from build123d import *

# Parameters (mm, degrees)
SKETCH4_W               = 63.691174053
SKETCH4_H               = 96.012068348
CUT_EXTRUDE3_DEPTH      = 86.451740766
CUT_EXTRUDE4_DEPTH      = 86.451740766
CUT_EXTRUDE4_DEPTH_BACK = 86.451740766
SKETCH6_R               = 1.65
CUT_EXTRUDE5_DEPTH      = 90.173515588
CUT_EXTRUDE5_DEPTH_BACK = 90.173515588
SKETCH7_R               = 1.65
SKETCH9_R               = 1.65
CUT_EXTRUDE7_DEPTH      = 5
BOSS_EXTRUDE4_START     = 27
SKETCH16_R              = 3.65
SKETCH16_R_2            = 1.65
BOSS_EXTRUDE4_DEPTH     = 3.9
BOSS_EXTRUDE6_START     = -16
SKETCH17_R              = 3.65
SKETCH17_R_2            = 1.65
BOSS_EXTRUDE6_DEPTH     = 3.9
BOSS_EXTRUDE7_START     = 4
SKETCH18_R              = 1.65
BOSS_EXTRUDE7_DEPTH     = 4
CUT_EXTRUDE8_DEPTH      = 0.2
SKETCH22_R              = 2.05
BOSS_EXTRUDE8_DEPTH     = 2
MIRROR2_COPY_1_SKETCH_R = 2.05
MIRROR2_COPY_1_DEPTH    = 2


with BuildPart() as part:
    # Sketch1 → Revolve1 (revolve)
    with BuildSketch(Plane(origin=(0, 0, 0), x_dir=(0, 0, -1), z_dir=(1, 0, 0)), mode=Mode.PRIVATE) as revolve1_sk:
        with BuildLine():
            Line((0, 12), (0, 11))
            Line((0, 11), (2, 11))
            Line((2, 11), (2, 10.5))
            ThreePointArc((2, 10.5), (3.464466094, 14.035533906), (7, 15.5))
            Line((7, 15.5), (12, 15.5))
            Line((12, 15.5), (75, 15.5))
            ThreePointArc((75, 15.5), (78.535533906, 14.035533906), (80, 10.5))
            Line((80, 10.5), (80, 0))
            Line((80, 0), (82, 0))
            Line((82, 0), (82, 12))
            ThreePointArc((82, 12), (80.535533906, 15.535533906), (77, 17))
            Line((77, 17), (5, 17))
            ThreePointArc((5, 17), (1.464466094, 15.535533906), (0, 12))
        make_face()
    revolve(revolve1_sk.sketch.rotate(Axis((0, 0, 0), (0, 0, -1)), 180), axis=Axis((0, 0, 0), (0, 0, -1)))

    # Sketch4 → Cut-Extrude3 (cut, through all)
    with BuildSketch(Plane(origin=(0, 0, 0), x_dir=(1, 0, 0), z_dir=(0, 1, 0))):
        with Locations((-0.095061454, 42.091351984)):
            Rectangle(SKETCH4_W, SKETCH4_H)
    extrude(amount=CUT_EXTRUDE3_DEPTH, mode=Mode.SUBTRACT)

    # Sketch6 → Cut-Extrude4 (cut, two sides: drawn at the far end of the back side and taken through both)
    with BuildSketch(Plane(origin=(0, 0, 0), x_dir=(0.7071067811865477, 0.7071067811865475, 0), z_dir=(-0.7071067811865475, 0.7071067811865477, 0)).offset(-CUT_EXTRUDE4_DEPTH_BACK)):
        with Locations(Location((0, 41, 0), (0, 0, 180))):
            Circle(SKETCH6_R)
    extrude(amount=CUT_EXTRUDE4_DEPTH + CUT_EXTRUDE4_DEPTH_BACK, mode=Mode.SUBTRACT)

    # Sketch7 → Cut-Extrude5 (cut, two sides: drawn at the far end of the back side and taken through both)
    with BuildSketch(Plane(origin=(7.778174593, 7.778174593, 0), x_dir=(0, 0, 1), z_dir=(-0.7071067811865438, -0.7071067811865512, 0)).offset(-CUT_EXTRUDE5_DEPTH_BACK)):
        with Locations(Location((-41, 0, 0), (0, 0, 270))):
            Circle(SKETCH7_R)
    extrude(amount=CUT_EXTRUDE5_DEPTH + CUT_EXTRUDE5_DEPTH_BACK, mode=Mode.SUBTRACT)

    # Sketch9 → Cut-Extrude7 (cut)
    with BuildSketch(Plane(origin=(0, 0, -82), x_dir=(-1, 0, 0), z_dir=(0, 0, -1))):
        with Locations(Location((0, -10, 0), (0, 0, 90))):
            Circle(SKETCH9_R)
    extrude(amount=-CUT_EXTRUDE7_DEPTH, mode=Mode.SUBTRACT)

    # Sketch16 → Boss-Extrude4 (add)
    with BuildSketch(Plane(origin=(7.778174593, 7.778174593, 0), x_dir=(0, 0, 1), z_dir=(-0.7071067811865438, -0.7071067811865512, 0)).offset(BOSS_EXTRUDE4_START)):
        with Locations(Location((-41, 0, 0), (0, 0, 90))):
            Circle(SKETCH16_R)
        with Locations(Location((-41, 0, 0), (0, 0, 270))):
            Circle(SKETCH16_R_2, mode=Mode.SUBTRACT)
    extrude(amount=BOSS_EXTRUDE4_DEPTH)

    # Sketch17 → Boss-Extrude6 (add)
    with BuildSketch(Plane(origin=(0, 0, 0), x_dir=(0.7071067811865477, 0.7071067811865475, 0), z_dir=(-0.7071067811865475, 0.7071067811865477, 0)).offset(BOSS_EXTRUDE6_START)):
        with Locations(Location((0, 41, 0), (0, 0, 180))):
            Circle(SKETCH17_R)
        with Locations(Location((0, 41, 0), (0, 0, 180))):
            Circle(SKETCH17_R_2, mode=Mode.SUBTRACT)
    extrude(amount=-BOSS_EXTRUDE6_DEPTH)

    # Sketch18 → Boss-Extrude7 (add)
    with BuildSketch(Plane(origin=(0, 0, -82), x_dir=(-1, 0, 0), z_dir=(0, 0, -1)).offset(BOSS_EXTRUDE7_START)):
        with BuildLine():
            Line((-4.806077942, -8.559024607), (-9, 0))
            Line((-9, 0), (-6.25, 0))
            ThreePointArc((-6.25, 0), (-5.298097039, -2.298097039), (-3, -3.25))
            Line((-3, -3.25), (3, -3.25))
            ThreePointArc((3, -3.25), (5.298097039, -2.298097039), (6.25, 0))
            Line((6.25, 0), (9, 0))
            Line((9, 0), (4.806077942, -8.559024607))
            ThreePointArc((4.806077942, -8.559024607), (4.337052511, -9.685379412), (4.008689498, -10.860469933))
            ThreePointArc((4.008689498, -10.860469933), (0, -14.1), (-4.008689498, -10.860469933))
            ThreePointArc((-4.008689498, -10.860469933), (-4.337052511, -9.685379412), (-4.806077942, -8.559024607))
        make_face()
        with Locations(Location((0, -10, 0), (0, 0, 90))):
            Circle(SKETCH18_R, mode=Mode.SUBTRACT)
    extrude(amount=-BOSS_EXTRUDE7_DEPTH)

    # Sketch20 → Cut-Extrude8 (cut)
    with BuildSketch(Plane(origin=(0, 0, -86), x_dir=(-1, 0, 0), z_dir=(0, 0, -1))):
        Polygon((-3.746989388, -4.234271569), (-3.1811841, -4.234271569), (-1.593143234, -6.537456665), (-1.593143234, -4.234271569), (-0.964938106, -4.234271569), (-0.964938106, -7.734271569), (-1.534950125, -7.734271569), (-3.11878426, -5.438097691), (-3.11878426, -7.734271569), (-3.746989388, -7.734271569), align=None)
        Polygon((-0.157245798, -4.234271569), (0.47095933, -4.234271569), (0.47095933, -7.106066441), (1.458138817, -7.106066441), (1.458138817, -7.734271569), (-0.157245798, -7.734271569), align=None)
        Polygon((1.996600356, -4.234271569), (3.88121574, -4.234271569), (3.88121574, -4.862476697), (2.624805484, -4.862476697), (2.624805484, -5.53555362), (3.88121574, -5.53555362), (3.88121574, -6.163758749), (2.624805484, -6.163758749), (2.624805484, -7.106066441), (3.88121574, -7.106066441), (3.88121574, -7.734271569), (1.996600356, -7.734271569), align=None)
    extrude(amount=-CUT_EXTRUDE8_DEPTH, mode=Mode.SUBTRACT)

    # Sketch22 → Boss-Extrude8 (add)
    with BuildSketch(Plane(origin=(0, 0, 0), x_dir=(1, 0, 0), z_dir=(0, 1, 0))):
        with BuildLine():
            Line((-17, 56.5), (-24.5, 56.5))
            ThreePointArc((-24.5, 56.5), (-26.267766953, 57.232233047), (-27, 59))
            Line((-27, 59), (-27, 65))
            ThreePointArc((-27, 65), (-26.267766953, 66.767766953), (-24.5, 67.5))
            Line((-24.5, 67.5), (-17, 67.5))
            Line((-17, 67.5), (-16.25, 67.5))
            Line((-16.25, 67.5), (-16.25, 56.5))
            Line((-16.25, 56.5), (-17, 56.5))
        make_face()
        with Locations(Location((-22, 62, 0), (0, 0, 270))):
            Circle(SKETCH22_R, mode=Mode.SUBTRACT)
    boss_extrude8 = extrude(amount=-BOSS_EXTRUDE8_DEPTH)

    # Mirror1: Boss-Extrude8 across plane
    add(boss_extrude8.mirror(Plane(origin=(0, 0, 0), x_dir=(0, 0, 1), z_dir=(1, 0, 0))))

    # Mirror2: Boss-Extrude8 across plane
    add(boss_extrude8.mirror(Plane(origin=(0, 0, -42.65), x_dir=(1, 0, 0), z_dir=(0, 0, -1))))

    # Mirror2 copy 1 sketch → Mirror2 copy 1 (add)
    with BuildSketch(Plane(origin=(0, 0, -85.3), x_dir=(-1, 0, 0), z_dir=(0, 1, 0))):
        with BuildLine():
            Line((-17, 56.5), (-24.5, 56.5))
            ThreePointArc((-24.5, 56.5), (-26.267766953, 57.232233047), (-27, 59))
            Line((-27, 59), (-27, 65))
            ThreePointArc((-27, 65), (-26.267766953, 66.767766953), (-24.5, 67.5))
            Line((-24.5, 67.5), (-17, 67.5))
            Line((-17, 67.5), (-16.25, 67.5))
            Line((-16.25, 67.5), (-16.25, 56.5))
            Line((-16.25, 56.5), (-17, 56.5))
        make_face()
        with Locations(Location((-22, 62, 0), (0, 0, 270))):
            Circle(MIRROR2_COPY_1_SKETCH_R, mode=Mode.SUBTRACT)
    extrude(amount=-MIRROR2_COPY_1_DEPTH)


solid = part.part
Input: part model. Units: mm. Frame: model coordinates. A direction names the side the tool comes from. Give positions to 0.01 mm unless a question says otherwise; leave off trailing zeros. Write each loop counter-clockwise with the first axis right and the second up, starting at its lowest first coordinate (ties: lowest second). Pieces come first, ordered by that corner, then holes.
Q1. Pull-direction query (Y, two-part tool) for faces 1 (the face through (-4.343, -9.669, -84.028)), 2 (the face through (-12.329, -13.448, -37.437)), 3 (the face through (-0.1, -13.3, -82)), 4 (the face through (-21, -1, -28.8)); classes: pulls with the +Y half, pulls with the -Y half, needs draft (parallel to the pull), parting line crosses it, or undercut.
Q2. Material intervals for probe 1 along X at (y, z) = (-0.45, -62); probe 2 along Z at (x, y) = (22, -0.6); probe 3 along Y at (x, z) = (0, -82.5), sorted ascending.
Q3. Section A-A, the plane z = -62. Output: boundary loops of the cut face in (x, y), plus the area to 3 significant figures.
Q4. Section C-C, the plane z = -32. Output: boundary loops of the cut face in (x, y).
Q5. First-contact query: P1, Ø1.6, axis at x = 21.5, y = -1, coming from the +Z side; P2, Ø4.5, axis at x = 22, z = -23.3, coming from the +Y side; P3, Ø5, axis at x = -13.5, y = -5, coming from the -Z side; P4, Ø10, axis at x = -18, y = -4, coming from the -Z side. Flat tips, straight axial feed; report the tip coordinate or a pass-through.
Q6. Set-up query: faces 5 (the face through (26.248, -0.986, -28.087)), 6 (the face through (-8, -6, -82)), 7 (the face through (-26.248, -0.986, -28.087)), 8 (the face through (4.33, -9.7, -84.03)), 9 (the face through (26.287, -0.986, -18.552)). Return all of +Z, -Z, +X, -X, +Y, -Y with unobstructed straight access to the full face (end or side cutting, diameter ignored); none if empty.
Q7. Section B-B, the plane x = 22. Output: boundary loops of the cut face in (y, z).
Filled in:
1. face 1: pulls with the -Y half
1. face 2: undercut
1. face 3: undercut
1. face 4: needs draft
2. probe 1: x = -27 to -24.05, -19.95 to -15.49, 15.49 to 19.95, 24.05 to 27
2. probe 2: z = -67.5 to -64.05, -59.95 to -56.5, -28.8 to -25.35, -21.25 to -17.8
2. probe 3: y = -14.1 to -11.65, -8.35 to -3.25
3. outline: (-27, -2) - (-24.05, -2) - (-24.05, 0) - (-27, 0) - close; (-19.95, -2) - (-16.88, -2) arc R17 ccw to (16.88, -2) - (19.95, -2) - (19.95, 0) - (15.5, 0) arc R15.5 cw to (-15.5, 0) - (-19.95, 0) - close; (24.05, -2) - (27, -2) - (27, 0) - (24.05, 0) - close
3. area: 100 mm2
4. outline: (-17, 0) arc R17 ccw to (17, 0) - (15.5, 0) arc R15.5 cw to (-15.5, 0) - close
5. P1: stops at z = -17.8
5. P2: stops at y = 0
5. P3: stops at z = -82
5. P4: stops at z = -81.79
6. face 5: +X, +Y, -Y
6. face 6: -Z, -X, -Y
6. face 7: -X, +Y, -Y
6. face 8: -Z, +X, -Y
6. face 9: +Z, +X, +Y, -Y
7. outline: (-2, -67.5) - (0, -67.5) - (0, -64.05) - (-2, -64.05) - close; (-2, -59.95) - (0, -59.95) - (0, -56.5) - (-2, -56.5) - close; (-2, -28.8) - (0, -28.8) - (0, -25.35) - (-2, -25.35) - close; (-2, -21.25) - (0, -21.25) - (0, -17.8) - (-2, -17.8) - close
